Source: CAD feature listing. Evaluate the final solid. Frame: model axes, mm. Face numbers are marked on the shaded views. A direction names the side the tool comes from. Coordinates: 2 decimals unless noted, no trailing zeros. Loops run counter-clockwise (first coordinate to the right, second up) from the corner with the lowest first, then second, coordinate; pieces in that order, holes last.
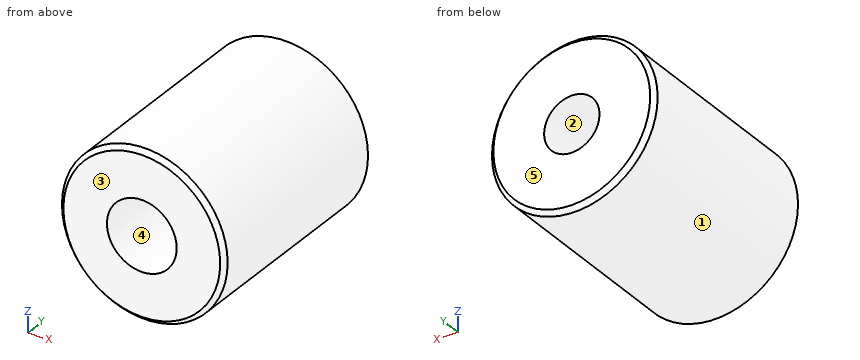
from build123d import *

# Parameters (mm, degrees)
F0_R     = 9.5
F0_R_2   = 3.175
F1_DEPTH = 24.7
F2_R     = 4
F3_DEPTH = 17
F4_SIZE  = 0.508


with BuildPart() as f1:
    # F0 (on Front) → F1 (new body)
    with BuildSketch(Plane.XZ):
        Circle(F0_R)
        Circle(F0_R_2, mode=Mode.SUBTRACT)
    extrude(amount=F1_DEPTH)

    # F2 (on face) → F3 (cut)
    with BuildSketch(Plane.XZ.offset(24.7)):
        Circle(F2_R)
    extrude(amount=-F3_DEPTH, mode=Mode.SUBTRACT)

    # F4
    f4_edges = [f1.edges().sort_by_distance(p)[0] for p in [
        (9.5, -12.35, 0),
        (-9.5, 0, 0),
        (-9.5, -24.7, 0),
    ]]
    chamfer(f4_edges, length=F4_SIZE)


solid = f1.part
Q1. Draft query along Z for the marked faces 1, 2 and 3. Return one class per face: +Z half, -Z half, draft (parallel to the pull), parting line (faces both ways), or undercut.
Q2. Section A-A, the plane z = 0. Return the cut outline in (x, y) (3 decimals), plus the area to 3 significant figures.
Q3. Section D-D, the plane y = -10.25. Return the cut outline in (x, z), plus the area to 3 significant figures.
Q4. Contact query for flat-ended pins moving along their axis: pin 1 Ø5.5 at (x, z) = (0, 0) entering from -Y; pin 2 Ø4 at (x, z) = (-1.5, -1) entering from -Y; pin 3 Ø3 at (x, y) = (7, -5) entering from +Z; pin 4 Ø2 at (y, z) = (-6.5, -6) entering from +X. Output: stop coordinate, or through.
Q5. Access query for the marked faces 4 and 5. Directions: +Z, -Z, +X, -X, +Y, -Y. A direction counts if a zero-diameter tool reaches every point of the face in a straight line with its end or side. Return the directions, or none.
Q6. Section B-B, the plane x = 0. Return the cut outline in (y, z) (3 decimals).
Q7. Line query: line 1 along Z through (x, y) = (0, -16.25); line 2 along Z through (x, y) = (0, -4) (3 decimals); line 3 along X through (y, z) = (-13.5, 3.5). Output: solid intervals per line, ascending.
Q8. Section C-C, the plane y = -3.75. Return the cut outline in (x, z) (3 decimals), plus the area to 3 significant figures.
Derived:
1. face 1: parting line
1. face 2: undercut
1. face 3: draft
2. outline: (-9.5, -24.192) - (-8.992, -24.7) - (-4, -24.7) - (-4, -7.7) - (-3.175, -7.7) - (-3.175, 0) - (-8.992, 0) - (-9.5, -0.508) - close; (3.175, -7.7) - (4, -7.7) - (4, -24.7) - (8.992, -24.7) - (9.5, -24.192) - (9.5, -0.508) - (8.992, 0) - (3.175, 0) - close
2. area: 284 mm2
3. outline: circle Ø19 at (0, 0); hole circle Ø8 at (0, 0)
3. area: 233 mm2
4. pin 1: passes through
4. pin 2: stops at y = -7.7
4. pin 3: stops at z = 7.75
4. pin 4: stops at x = 8.08
5. face 4: -Y
5. face 5: +Z, -Z, +X, -X, +Y
6. outline: (-24.7, -8.992) - (-24.192, -9.5) - (-0.508, -9.5) - (0, -8.992) - (0, -3.175) - (-7.7, -3.175) - (-7.7, -4) - (-24.7, -4) - close; (-24.7, 4) - (-7.7, 4) - (-7.7, 3.175) - (0, 3.175) - (0, 8.992) - (-0.508, 9.5) - (-24.192, 9.5) - (-24.7, 8.992) - close
7. line 1: z = -9.5 to -4, 4 to 9.5
7. line 2: z = -9.5 to -3.175, 3.175 to 9.5
7. line 3: x = -8.83 to -1.94, 1.94 to 8.83
8. outline: circle Ø19 at (0, 0); hole circle Ø6.35 at (0, 0)
8. area: 252 mm2
